```python
from build123d import *

# Parameters (mm, degrees)
SKETCH1_R           = 50
BOSS_EXTRUDE1_DEPTH = 112.5
SKETCH2_W           = 75
SKETCH2_H           = 300
SKETCH2_W_2         = 100
SKETCH2_H_2         = 75
CUT_EXTRUDE2_DEPTH  = 553.40949485


with BuildPart() as part:
    # Sketch1 → Boss-Extrude1 (new body)
    with BuildSketch(Plane.YZ):
        with BuildLine():
            Line((0, 150), (450, 150))
            Line((450, 150), (450, 75))
            Line((450, 75), (375, 75))
            Line((375, 75), (375, 100))
            Line((375, 100), (250, 100))
            Line((250, 100), (250, -100))
            Line((250, -100), (375, -100))
            Line((375, -100), (375, -25))
            Line((375, -25), (450, -25))
            Line((450, -25), (450, -150))
            Line((450, -150), (0, -150))
            ThreePointArc((0, -150), (-150, 0), (0, 150))
        make_face()
        with Locations(Location((0, 0, 0), (0, 0, 270))):
            Circle(SKETCH1_R, mode=Mode.SUBTRACT)
    extrude(amount=BOSS_EXTRUDE1_DEPTH)

    # Mirror1: part across plane


with BuildPart() as part_1:
    add(part.part)
    add(part.part.mirror(Plane(origin=(0, 0, 0), x_dir=(0, 0, 1), z_dir=(1, 0, 0))))

    # Sketch2 → Cut-Extrude2 (cut, through all)
    with BuildSketch(Plane.XY.offset(150)):
        with Locations((75, 0)):
            Rectangle(SKETCH2_W, SKETCH2_H)
        with Locations((62.5, 412.5)):
            Rectangle(SKETCH2_W_2, SKETCH2_H_2)
        with Locations((-75, 0)):
            Rectangle(SKETCH2_W, SKETCH2_H)
        with Locations((-62.5, 412.5)):
            Rectangle(SKETCH2_W_2, SKETCH2_H_2)
    extrude(amount=-CUT_EXTRUDE2_DEPTH, mode=Mode.SUBTRACT)


solid = part_1.part
```
Input: part model. Units: mm. Frame: model coordinates. A direction names the side the tool comes from. Round coordinates to 2 decimals unless told otherwise and drop trailing zeros. Loops run counter-clockwise (first coordinate to the right, second up) from the corner with the lowest first, then second, coordinate; pieces in that order, holes last. Notation, with made-up numbers: M 49,54 L 66,54 A19 cw 66,67 Z; hole C -33.75,89 d5. An arc over 180 degrees is marked long. Answer in a Markdown table with one row per item. Add a question column.
1. Ray query, probe 1 along Y at (x, z) = (17.5, 0); probe 2 along Z at (x, y) = (-14, 0); probe 3 along Y at (x, z) = (-85.5, -70). Return the intervals inside material, ascending.
2. Section A-A (y = 272). Output: boundary loops of the cut face in (x, z).
3. Section D-D (z = -107.5). Output: boundary loops of the cut face in (x, y), and give its area (3 significant figures).
4. Mould query, pull axis Z, two halves, no side actions, for faces 1 (the face through (-12.5, 412, -87)), 2 (the face through (2, 222, 150)), 3 (the face through (2, 312, -100)), 4 (the face through (2, 313, 100)). Classes: released by +Z, released by -Z, zero draft, split by the parting line, or undercut.
5. Section B-B (z = 0). Output: boundary loops of the cut face in (x, y), and give its area (3 significant figures).
6. Section C-C (x = 97). Output: boundary loops of the cut face in (y, z), and give its area (3 significant figures).
7. Contact query for flat-ended pins moving along their axis: pin 1 (12 mm diameter, centred on x = -89, z = -72.5, fed in from +Y); pin 2 (3 mm diameter, centred on y = -46.5, z = -78, fed in from +X); pin 3 (6 mm diameter, centred on x = -85.5, z = 30.5, fed in from -Y). Output: stop coordinate, or through.
8. Set-up query: faces 5 (the face through (-63, 375, 125)), 6 (the face through (62, 375, -125)), 7 (the face through (0, 412, -25)), 8 (the face through (-37.5, 65, 2)). Return all of +Z, -Z, +X, -X, +Y, -Y with unobstructed straight access to the full face (end or side cutting, diameter ignored); none if empty.
Values follow:
| question | item | result |
|---|---|---|
| 1 | probe 1 | -150 to -50, 50 to 250 |
| 1 | probe 2 | -150 to -50, 50 to 150 |
| 1 | probe 3 | 150 to 250 |
| 2 | outline | M -112.5,-150 L 112.5,-150 L 112.5,-100 L -112.5,-100 Z; M -112.5,100 L 112.5,100 L 112.5,150 L -112.5,150 Z |
| 3 | outline | M -112.5,150 L -37.5,150 L -37.5,-104.61 L 37.5,-104.61 L 37.5,150 L 112.5,150 L 112.5,375 L 12.5,375 L 12.5,450 L -12.5,450 L -12.5,375 L -112.5,375 Z |
| 3 | area | 71,600 mm^2 |
| 4 | face 1 | zero draft |
| 4 | face 2 | released by +Z |
| 4 | face 3 | undercut |
| 4 | face 4 | undercut |
| 5 | outline | M -112.5,150 L -37.5,150 L -37.5,50 L 37.5,50 L 37.5,150 L 112.5,150 L 112.5,250 L -112.5,250 Z; M -37.5,-150 L 37.5,-150 L 37.5,-50 L -37.5,-50 Z |
| 5 | area | 37,500 mm^2 |
| 6 | outline | M 150,-150 L 375,-150 L 375,-100 L 250,-100 L 250,100 L 375,100 L 375,150 L 150,150 Z |
| 6 | area | 42,500 mm^2 |
| 7 | pin 1 | y = 250 |
| 7 | pin 2 | x = 37.5 |
| 7 | pin 3 | y = 150 |
| 8 | face 5 | +Z, -Z, -X, +Y |
| 8 | face 6 | +Z, -Z, +X, +Y |
| 8 | face 7 | +X, -X, +Y |
| 8 | face 8 | +Z, -Z, -X, -Y |
